Could you check a few things on this model? Use its own coordinates, in mm. Face numbers are marked on the shaded views. A direction names the side the tool comes from. Give positions to 0.01 mm unless a question says otherwise; leave off trailing zeros. Write each loop counter-clockwise with the first axis right and the second up, starting at its lowest first coordinate (ties: lowest second). Pieces come first, ordered by that corner, then holes. Notation, with made-up numbers: (55, -11.75) - (85, -11.75) arc R29 ccw to (85, 16.25) - close; hole circle Ø7 at (-30, 74). An arc over 180 degrees is marked (long way). Write item = value, one per line.
from build123d import *

# Parameters (mm, degrees)
BOSS_EXTRUDE1_DEPTH      = 8
BOSS_EXTRUDE1_DEPTH_BACK = 8
SKETCH2_R                = 100
CUT_EXTRUDE1_DEPTH       = 3
CUT_EXTRUDE1_DEPTH_BACK  = 3
SKETCH2_5_R              = 100
SKETCH2_5_R_2            = 98
LPATTERN1_COUNT          = 2
LPATTERN1_PITCH          = 76
SKETCH5_W                = 140
SKETCH5_H                = 60
SKETCH5_R                = 3.2
BOSS_EXTRUDE2_DEPTH      = 30
SKETCH7_R                = 4.5
SKETCH7_R_2              = 3.4
SKETCH7_R_3              = 5
CUT_EXTRUDE2_DEPTH       = 167
SKETCH3_R                = 33.75
CUT_EXTRUDE3_DEPTH       = 43
SKETCH10_R               = 6
BOSS_EXTRUDE3_DEPTH      = 60
CUT_EXTRUDE4_DEPTH       = 112
CUT_EXTRUDE4_DEPTH_BACK  = 60
SKETCH10_4_R             = 4.5
SKETCH11_R               = 10
CUT_EXTRUDE5_DEPTH       = 60


with BuildPart() as part:
    # Sketch2 → Boss-Extrude1 (new, two sides: drawn at the far end of the back side and taken through both)
    with BuildSketch(Plane.XY.offset(-BOSS_EXTRUDE1_DEPTH_BACK)):
        Circle(SKETCH2_R)
    extrude(amount=BOSS_EXTRUDE1_DEPTH + BOSS_EXTRUDE1_DEPTH_BACK)

    # Sketch2_5 → Cut-Extrude1 (cut, two sides: drawn at the far end of the back side and taken through both)
    with BuildSketch(Plane.XY.offset(-CUT_EXTRUDE1_DEPTH_BACK)):
        Circle(SKETCH2_5_R)
        Circle(SKETCH2_5_R_2, mode=Mode.SUBTRACT)
    extrude(amount=CUT_EXTRUDE1_DEPTH + CUT_EXTRUDE1_DEPTH_BACK, mode=Mode.SUBTRACT)


with BuildPart() as lpattern1_1:
    # LPattern1: pattern copy
    add(part.part.moved(Location(Vector(0, 0, -1) * (1 * LPATTERN1_PITCH))))


with BuildPart() as part_1:
    add(part.part)

    # Sketch5 → Boss-Extrude2 (add)
    with BuildSketch(Plane(origin=(0, -33.75, 0), x_dir=(1, 0, 0), z_dir=(0, 1, 0))):
        with Locations((0, 38)):
            Rectangle(SKETCH5_W, SKETCH5_H)
        with Locations(Location((0, 43, 0), (0, 0, 180))):
            Circle(SKETCH5_R, mode=Mode.SUBTRACT)
    extrude(amount=-BOSS_EXTRUDE2_DEPTH)


with BuildPart() as cut_extrude2_tool:
    # Sketch7 → Cut-Extrude2 (new body)
    with BuildSketch(Plane.XY.offset(8)):
        with Locations((-50, -48.75)):
            Circle(SKETCH7_R)
        with Locations((50, -48.75)):
            Circle(SKETCH7_R)
        with Locations((-20, -48.75)):
            Circle(SKETCH7_R_2)
        with Locations((20, -48.75)):
            Circle(SKETCH7_R_3)
    extrude(amount=-CUT_EXTRUDE2_DEPTH)


with BuildPart() as part_2:
    add(part_1.part)

    # Cut-Extrude2: cut by cut_extrude2_tool
    add(cut_extrude2_tool.part, mode=Mode.SUBTRACT)

    # Sketch3 → Cut-Extrude3 (cut)
    with BuildSketch(Plane.XY.offset(8)):
        Circle(SKETCH3_R)
    extrude(amount=-CUT_EXTRUDE3_DEPTH, mode=Mode.SUBTRACT)



with BuildPart() as lpattern1_1_1:
    add(lpattern1_1.part)

    # Cut-Extrude2: cut by cut_extrude2_tool
    add(cut_extrude2_tool.part, mode=Mode.SUBTRACT)


with BuildPart() as part_3:
    add(part_2.part)

    add(lpattern1_1_1.part)  # Boss-Extrude3 merges LPattern1_1
    # Sketch10 → Boss-Extrude3 (add)
    with BuildSketch(Plane(origin=(0, 0, -8), x_dir=(-1, 0, 0), z_dir=(0, 0, -1))):
        with Locations(Location((0, 70, 0), (0, 0, 180))):
            Circle(SKETCH10_R)
    extrude(amount=BOSS_EXTRUDE3_DEPTH)

    # Sketch10_4 → Cut-Extrude4 (cut, two sides: drawn at the far end of the back side and taken through both)
    with BuildSketch(Plane(origin=(0, 0, -8), x_dir=(-1, 0, 0), z_dir=(0, 0, -1)).offset(-CUT_EXTRUDE4_DEPTH_BACK)):
        with Locations(Location((0, 70, 0), (0, 0, 180))):
            Circle(SKETCH10_4_R)
    extrude(amount=CUT_EXTRUDE4_DEPTH + CUT_EXTRUDE4_DEPTH_BACK, mode=Mode.SUBTRACT)

    # Sketch11 → Cut-Extrude5 (cut)
    with BuildSketch(Plane(origin=(0, 0, -84), x_dir=(-1, 0, 0), z_dir=(0, 0, -1))):
        with Locations((-45, -15)):
            Circle(SKETCH11_R)
    extrude(amount=-CUT_EXTRUDE5_DEPTH, mode=Mode.SUBTRACT)


solid = part_3.part
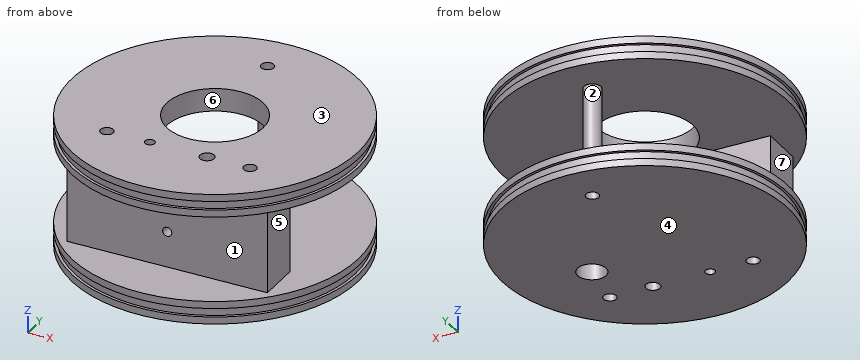
1. For pin 1 (24 mm diameter, centred on y = -50, z = -40.5, fed in from +X); pin 2 (15 mm diameter, centred on y = -52, z = -27.5, fed in from -X); pin 3 (8 mm diameter, centred on x = -69, z = -52.5, fed in from -Y); pin 4 (11.5 mm diameter, centred on x = 0, y = 70, fed in from -Z), each with a flat end and sliding along its axis, tell me the tip position at first contact or that it passes through.
Filled sheet:
pin_1 = 70
pin_2 = -70
pin_3 = -63.75
pin_4 = -84
2. Which directions (+Z, -Z, +X, -X, +Y, -Y) give clear straight access to the entire face, cutting with the end or side of a thin tool? Please do the marked faces 4, 5, 6 and 7.
Filled sheet:
face_4 = -Z, +X, -X, +Y, -Y
face_5 = +X, +Y, -Y
face_6 = +Z
face_7 = -X, +Y, -Y
3. Thinking about a two-plate mould opening in Y: for the marked faces 1, 2 and 3, which applies, pulls with the +Y half, pulls with the -Y half, needs draft (parallel to the pull), parting line crosses it, or undercut?
Filled sheet:
face_1 = pulls with the -Y half
face_2 = undercut
face_3 = needs draft
4. If we section it at B-B, the plane y = -11: Count the separate pieces of the cut face and the enclosed holes in it, and give its area (3 significant figures).
Filled sheet:
separate_pieces = 4
enclosed_holes = 0
area = 5,000 mm2
5. I need wall thicknesses on line 1 (Y direction, x = 0, z = -4); line 2 (Y direction, x = 0, z = 0); line 3 (Z direction, x = -28.5, y = 21). Which ranges of each line are inside material? Lowest first, please.
Filled sheet:
line_1 = -100 to -33.75, 33.75 to 65.5, 74.5 to 100
line_2 = -98 to -33.75, 33.75 to 65.5, 74.5 to 98
line_3 = -84 to -68, -8 to 8
6. If we section it at A-A, the plane z = -50: Please give me the cut outline in (x, y).
Filled sheet:
outline = (-70, -63.75) - (70, -63.75) - (70, -33.75) - (-70, -33.75) - close; circle Ø12 at (0, 70); hole circle Ø9 at (-50, -48.75); hole circle Ø6.8 at (-20, -48.75); hole circle Ø9 at (0, 70); hole circle Ø10 at (20, -48.75); hole circle Ø9 at (50, -48.75)
7. If we section it at D-D, the plane y = -68: Please give me the cut outline in (x, z), and give its area (3 significant figures).
Filled sheet:
outline = (-73.32, -84) - (73.32, -84) - (73.32, -79) - (70.57, -79) - (70.57, -73) - (73.32, -73) - (73.32, -68) - (-73.32, -68) - (-73.32, -73) - (-70.57, -73) - (-70.57, -79) - (-73.32, -79) - close; (-73.32, -8) - (73.32, -8) - (73.32, -3) - (70.57, -3) - (70.57, 3) - (73.32, 3) - (73.32, 8) - (-73.32, 8) - (-73.32, 3) - (-70.57, 3) - (-70.57, -3) - (-73.32, -3) - close
area = 4,630 mm2
